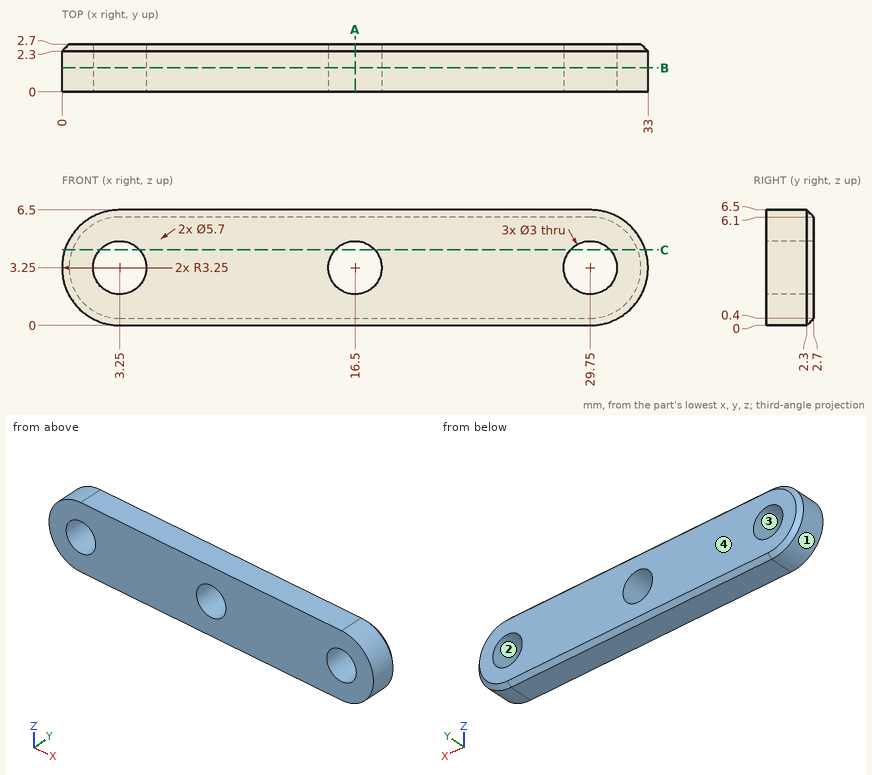
Job drawing, mm, ordinate dimensions from the low corner. One solid piece. Round coordinates to 2 decimals unless told otherwise and drop trailing zeros. Loops run counter-clockwise (first coordinate to the right, second up) from the corner with the lowest first, then second, coordinate; pieces in that order, holes last. Notation, with made-up numbers: (0, 3) -> (5, 3) arc R15 ccw to (5, 13) -> close; hole circle Ø8 at (-4, -19.75). An arc over 180 degrees is marked (long way). One line per item, written item: value. Start each with the question number.
Q1. Two-plate mould, pull along Z, no slides. Class the marked faces 1, 2, 3 and 4: released by +Z, released by -Z, zero draft, split by the parting line, or undercut.
Q2. Cut at B-B on y = 1.35. List the corners of the cut face in (x, z).
Q3. Probe line 1 along X through (y, z) = (1.8, 3.25); line 2 along X through (y, z) = (0.8, 2.5); line 3 along Z through (x, y) = (29.75, 1.65). List the from-to ranges inside material, lowest first.
Q4. Cut at A-A on x = 16.5. List the corners of the cut face in (y, z).
Q5. Drop a flat-ended pin along its axis: pin 1 Ø2.5 at (x, z) = (29.75, 3.25) entering from -Y. Give the stop position or say it passes through.
Q6. Cut at C-C on z = 4.25. Count the separate pieces of the cut face and the enclosed holes in it, plus the area to 3 significant figures.
Computed:
1. face 1: split by the parting line
1. face 2: undercut
1. face 3: undercut
1. face 4: zero draft
2. outline: (3.25, 0) -> (29.75, 0) arc R3.25 ccw to (29.75, 6.5) -> (3.25, 6.5) arc R3.25 ccw to start; hole circle Ø3 at (3.25, 3.25); hole circle Ø3 at (16.5, 3.25); hole circle Ø3 at (29.75, 3.25)
3. line 1: 0 to 1.75, 4.75 to 15, 18 to 28.25, 31.25 to 33
3. line 2: 0.09 to 1.95, 4.55 to 15.2, 17.8 to 28.45, 31.05 to 32.91
3. line 3: 0 to 1.75, 4.75 to 6.5
4. outline: (0, 0) -> (2.3, 0) -> (2.7, 0.4) -> (2.7, 1.75) -> (0, 1.75) -> close; (0, 4.75) -> (2.7, 4.75) -> (2.7, 6.1) -> (2.3, 6.5) -> (0, 6.5) -> close
5. pin 1: through
6. separate pieces: 4
6. enclosed holes: 0
6. area: 70.0 mm²
